Check sheet for the modelled part. Datum: model origin and axes. Units: mm. A direction names the side the tool comes from. Give positions to 0.01 mm unless a question says otherwise; leave off trailing zeros. Loops run counter-clockwise (first coordinate to the right, second up) from the corner with the lowest first, then second, coordinate; pieces in that order, holes last. Notation, with made-up numbers: (-17, 26) -> (14, 26) arc R16 ccw to (14, 56) -> close; hole circle Ø10 at (10.25, -5.5). An arc over 180 degrees is marked (long way). Write each question's results on one line, items separated by ' | '. Start each with the question number.
Item 1: Cross-section at C-C on z = 15. Enter the section's corners in (x, y), then the cut area to 3 significant figures.
Item 2: Access from +Z, -Z, +X, -X, +Y, -Y to the whole of each face (thin tool, end or side, straight path). Record for faces 1 (the face through (-19.85, 19.6, 1.97)), 2 (the face through (2, -18, 2.75)), 3 (the face through (-2, -18, 2.75)), 4 (the face through (45, 27, 7)).
Item 3: Scan lines: line 1 along X through (y, z) = (-8.5, 1.75); line 2 along Z through (x, y) = (-26, 17.5); line 3 along Y through (x, z) = (41, 14.5). Record each from-to range of solid material in increasing order.
Item 4: Mould release check, pull along X, two halves, no side actions. Record for faces 5 (the face through (19.85, 19.6, 1.97)), 6 (the face through (0.1, -7.5, 3.7)), 7 (the face through (-4, 8, 0)), 8 (the face through (-0.015, 7.842, 2.028)): pulls with the +X half, pulls with the -X half, needs draft (parallel to the pull), parting line crosses it, or undercut.
Item 5: Cross-section at A-A on y = 13.5. Enter the section's corners in (x, z).
Item 6: Cross-section at B-B on y = -14.5. Enter the section's corners in (x, z), then the cut area to 3 significant figures.
Item 7: Cross-section at D-D on x = -31. Enter the section's corners in (y, z).
Item 8: Gauge pin test, flat ends, axial feed: pin 1 Ø6 at (x, y) = (3.5, 1.5) entering from +Z; pin 2 Ø5 at (x, z) = (2.5, 8) entering from +Y; pin 3 Ø1.9 at (x, y) = (1, -23) entering from -Z; pin 4 Ø0.5 at (x, y) = (-1.5, -23) entering from -Z. Record the tip position at first contact, or that the pin passes through.
Autodesk Inventor part; units mm, degrees
ref_plane "YZ Plane" through (0, 0, 0) normal (1, 0, 0) x (0, 1, 0)
ref_plane "XZ Plane" through (0, 0, 0) normal (0, 1, 0) x (-1, 0, 0)
ref_plane "XY Plane" through (0, 0, 0) normal (0, 0, 1) x (1, 0, 0)
sketch "Sketch1" plane through (0, 0, 0) normal (0, 0, 1) x (1, 0, 0)
  arc A0 (44.3036, 23.0175) -> (39.2001, 31.3912) centre (42.588, 27.714) ccw
  arc A1 (-39.2001, 31.3912) -> (-44.3036, 23.0175) centre (-42.588, 27.714) ccw
  arc A2 (-6.666, -3.4373) -> (6.666, -3.4373) centre (0, 0) ccw
  line L0 (0, 7.5) -> (39.2001, 31.3912)
  line L1 (6.666, -3.4373) -> (44.3036, 23.0175)
  line L2 (0, 7.5) -> (-39.2001, 31.3912)
  line L3 (-6.666, -3.4373) -> (-44.3036, 23.0175)
  dimension "d5" = 10
  dimension "d6" = 10
  dimension "d7" = 15
extrude "Extrusion1" add sketch "Sketch1" along normal blind 4
fillet "Fillet1" radius 2 1 edges at (0, 7.5, 2)
sketch "Sketch2" plane through (0, 0, 4) normal (0, 0, 1) x (1, 0, 0)
  arc A0 (44.3036, 23.0175) -> (39.2001, 31.3912) centre (42.588, 27.714) ccw
  circle A1 centre (42.588, 27.714) radius 2.25
  arc A2 (-39.2001, 31.3912) -> (-44.3036, 23.0175) centre (-42.588, 27.714) ccw
  circle A3 centre (-42.588, 27.714) radius 2.25
  point P0 (0, 0)
  dimension "d11" = 4.5
  dimension "d12" = 4.5
extrude "Extrusion2" add sketch "Sketch2" along normal blind 12
sketch "Sketch3" plane through (0, 0, 4) normal (0, 0, 1) x (1, 0, 0)
  arc A0 (44.3036, 23.0175) -> (39.2001, 31.3912) centre (42.588, 27.714) ccw
  circle A1 centre (42.588, 27.714) radius 2.75
  circle A2 centre (-42.588, 27.714) radius 2.25
  circle A3 centre (-42.588, 27.714) radius 2.75
  point P0 (0, 0)
  dimension "d15" = 5.5
  dimension "d16" = 5.5
extrude "Extrusion3" add sketch "Sketch3" along normal blind 3 contours A1 | A2 | A3
sketch "Sketch4" plane through (0, 0, 0) normal (0, 1, 0) x (-1, 0, 0)
  line L0 (2.5, 1.25) -> (-2.5, 1.25)
  line L1 (-2.5, 1.25) -> (-2.5, 2.75)
  line L2 (-2.5, 2.75) -> (2.5, 2.75)
  line L3 (2.5, 2.75) -> (2.5, 1.25)
  line L4 (2.5, 1.25) -> (-2.5, 2.75) construction
  line L5 (-2.5, 1.25) -> (2.5, 2.75) construction
  line L6 (-0.75, 0.5) -> (-0.75, 3.5)
  line L7 (-0.75, 3.5) -> (0.75, 3.5)
  line L8 (0.75, 3.5) -> (0.75, 0.5)
  line L9 (0.75, 0.5) -> (-0.75, 0.5)
  line L10 (-0.75, 0.5) -> (0.75, 3.5) construction
  line L11 (-0.75, 3.5) -> (0.75, 0.5) construction
  point P0 (0, 0)
  point P1 (0, 2)
  point P2 (0, 2)
  point P3 (-0.75, 2.75)
  point P4 (-0.75, 1.25)
  point P5 (0.75, 1.25)
  point P6 (0.75, 2.75)
  dimension "d19" = 5
  dimension "d20" = 1.5
  dimension "d21" = 3
  dimension "d22" = 1.5
extrude "Extrusion4" add sketch "Sketch4" against normal blind 30
sketch "Sketch5" plane through (0, 0, 4) normal (0, 0, 1) x (1, 0, 0)
  point P0 (0, 0)
sketch "Sketch6" plane through (0, -30, 0) normal (0, -1, 0) x (1, 0, 0)
  point P0 (0, 0)
properties part number "Gripper Base" material "Gold"
Answer sheet:
1) outline: circle Ø4.5 at (-42.59, 27.71); circle Ø4.5 at (42.59, 27.71) | area: 31.8 mm²
2) face 1: +Z, -Z, +Y | face 2: +Z, +X, -Y | face 3: +Z, -X, -Y | face 4: +Z
3) line 1: x = -2.5 to 2.5 | line 2: z = 0 to 4 | line 3: y = 26.12 to 29.31
4) face 5: undercut | face 6: parting line crosses it | face 7: needs draft | face 8: undercut
5) outline: (-30.76, 0) -> (-9.84, 0) -> (-9.84, 4) -> (-30.76, 4) -> close; (9.84, 0) -> (30.76, 0) -> (30.76, 4) -> (9.84, 4) -> close
6) outline: (-2.5, 1.25) -> (-0.75, 1.25) -> (-0.75, 0.5) -> (0.75, 0.5) -> (0.75, 1.25) -> (2.5, 1.25) -> (2.5, 2.75) -> (0.75, 2.75) -> (0.75, 3.5) -> (-0.75, 3.5) -> (-0.75, 2.75) -> (-2.5, 2.75) -> close | area: 9.75 mm²
7) outline: (13.67, 0) -> (26.39, 0) -> (26.39, 4) -> (13.67, 4) -> close
8) pin 1: stops at z = 4 | pin 2: passes through | pin 3: stops at z = 0.5 | pin 4: stops at z = 1.25
